Geometry check sheet. Reference: the model listing, model coordinates, mm. Face numbers are marked on the shaded views. A direction names the side the tool comes from. Coordinates: 2 decimals unless noted, no trailing zeros. Loops run counter-clockwise (first coordinate to the right, second up) from the corner with the lowest first, then second, coordinate; pieces in that order, holes last.
from build123d import *

# Parameters (mm, degrees)
MAIN_BODY_DEPTH          = 6.35
BATTERY_SPACING_DEPTH    = 2.54
SKETCH8_R                = 4.064
LIGHT_SOCKETS_DEPTH      = 12.7
LIGHT_LEADS_POCKET_DEPTH = 6.35
WIRE_TRAIL_DEPTH         = 2.54
LEAD_ROOM_DEPTH          = 7.62
FILLET1_R                = 7.62
TAB_SLOTS_DEPTH          = 1.778
SKETCH14_W               = 10.16
SKETCH14_H               = 6.35
SCREW_MOUNT_DEPTH        = 10.16


# Sheet-metal steps are written as plain solids
with BuildPart() as part:
    # Sketch1 → Main Body (new body)
    with BuildSketch(Plane.XY):
        Polygon((-53.975, 0), (53.975, 0), (57.15, 82.161327118), (101.6, 101.6), (101.6, 146.05), (-101.6, 146.05), (-101.6, 101.6), (-57.15, 82.161327118), align=None)
    extrude(amount=-MAIN_BODY_DEPTH)

    # Sketch7 → Battery Spacing (cut)
    with BuildSketch(Plane.XY):
        Polygon((-50.564894027, 76.2), (-47.86564661, 6.35), (47.86564661, 6.35), (50.564894027, 76.2), align=None)
    extrude(amount=-BATTERY_SPACING_DEPTH, mode=Mode.SUBTRACT)

    # Sketch8 → Light Sockets (cut)
    with BuildSketch(Plane.XY):
        with Locations((85.852, 123.825)):
            Circle(SKETCH8_R)
        with Locations((-85.852, 123.825)):
            Circle(SKETCH8_R)
        with BuildLine():
            Line((-5.969, 131.318), (5.969, 131.318))
            ThreePointArc((5.969, 131.318), (13.462, 123.825), (5.969, 116.332))
            Line((5.969, 116.332), (-5.969, 116.332))
            ThreePointArc((-5.969, 116.332), (-13.462, 123.825), (-5.969, 131.318))
        make_face()
    extrude(amount=-LIGHT_SOCKETS_DEPTH, mode=Mode.SUBTRACT)

    # Sketch9 → Light Leads Pocket (add)
    with BuildSketch(Plane(origin=(0, 0, -6.35), x_dir=(-1, 0, 0), z_dir=(0, 0, -1))):
        with BuildLine():
            Line((-9.525, 111.765348554), (-9.525, 99.065348554))
            Line((-9.525, 99.065348554), (9.525, 99.065348554))
            Line((9.525, 99.065348554), (9.525, 111.765348554))
            ThreePointArc((9.525, 111.765348554), (18.413001098, 125.621431375), (5.969, 136.398))
            Line((5.969, 136.398), (-5.969, 136.398))
            ThreePointArc((-5.969, 136.398), (-18.413001098, 125.621431375), (-9.525, 111.765348554))
        make_face()
    extrude(amount=LIGHT_LEADS_POCKET_DEPTH)

    # Sketch10 → Wire Trail (cut)
    with BuildSketch(Plane.XY):
        Polygon((-3.175, 116.332), (3.175, 116.332), (3.175, 76.2), (3.175, 6.35), (3.175, 0), (-3.175, 0), align=None)
    extrude(amount=-WIRE_TRAIL_DEPTH, mode=Mode.SUBTRACT)

    # Sketch12 → Lead Room (cut)
    with BuildSketch(Plane.XY.offset(-2.54)):
        with BuildLine():
            Line((-3.175, 116.332), (-5.960094489, 116.332))
            ThreePointArc((-5.960094489, 116.332), (-13.36178344, 123.73368895), (-5.960094489, 131.135377901))
            Line((-5.960094489, 131.135377901), (6.000168296, 131.135377901))
            ThreePointArc((6.000168296, 131.135377901), (13.401857247, 123.73368895), (6.000168296, 116.332))
            Line((6.000168296, 116.332), (3.175, 116.332))
            Line((3.175, 116.332), (3.175, 103.730451358))
            Line((3.175, 103.730451358), (-3.175, 103.730451358))
            Line((-3.175, 103.730451358), (-3.175, 116.332))
        make_face()
    extrude(amount=-LEAD_ROOM_DEPTH, mode=Mode.SUBTRACT)

    # Fillet1
    fillet1_edges = [part.edges().sort_by_distance(p)[0] for p in [
        (0, 103.730451358, -2.54),
    ]]
    fillet(fillet1_edges, radius=FILLET1_R - 0.0001)  # a hair under: the kernel refuses the full size

    # Sketch13 → Tab Slots (cut)
    with BuildSketch(Plane.XY):
        with BuildLine():
            Line((72.263, 146.05), (72.263, 123.825))
            ThreePointArc((72.263, 123.825), (85.852, 110.236), (99.441, 123.825))
            Line((99.441, 123.825), (99.441, 146.05))
            Line((99.441, 146.05), (72.263, 146.05))
        make_face()
    tab_slots = extrude(amount=-TAB_SLOTS_DEPTH, mode=Mode.SUBTRACT)

    # Mirror1: Tab Slots across plane
    add(tab_slots.mirror(Plane(origin=(0, 0, 0), x_dir=(0, 0, 1), z_dir=(1, 0, 0))), mode=Mode.SUBTRACT)

    # Sketch14 → Screw Mount (add)
    with BuildSketch(Plane.XZ):
        with Locations((48.895, -3.175)):
            Rectangle(SKETCH14_W, SKETCH14_H)
    screw_mount = extrude(amount=SCREW_MOUNT_DEPTH)

    # Mirror2: Screw Mount across plane
    add(screw_mount.mirror(Plane(origin=(0, 0, 0), x_dir=(0, 0, 1), z_dir=(1, 0, 0))))


solid = part.part
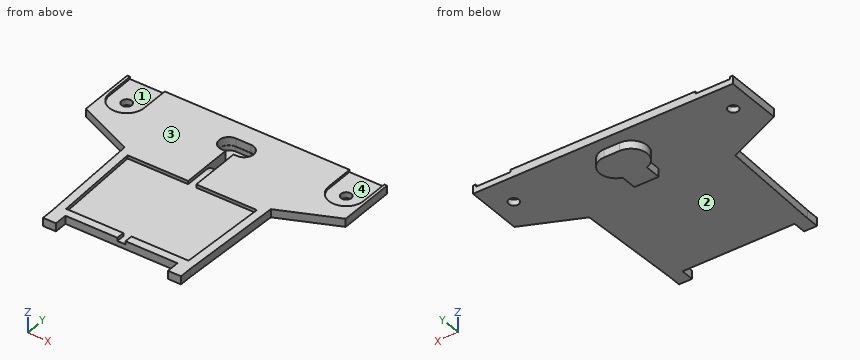
(1) Sectioned sample at C-C on x = -87. Record the cut outline in (y, z), and give its area (3 significant figures).
Findings:
outline: (95.22, -6.35) - (119.93, -6.35) - (119.93, -1.78) - (110.28, -1.78) - (110.28, 0) - (95.22, 0) - close; (127.72, -6.35) - (146.05, -6.35) - (146.05, -1.78) - (127.72, -1.78) - close
area: 224 mm2
(2) Sectioned sample at D-D on x = -24. Record the cut outline in (y, z).
Findings:
outline: (0, -6.35) - (146.05, -6.35) - (146.05, 0) - (76.2, 0) - (76.2, -2.54) - (6.35, -2.54) - (6.35, 0) - (0, 0) - close
(3) Draft check along X on the marked faces 1 and 2. Enter one of: +X half, -X half, draft (parallel to the pull), parting line (faces both ways), or undercut.
Findings:
face 1: undercut
face 2: draft
(4) Scan lines: L1, parallel to X at y = 127, z = -3; L2, parallel to Z at x = 7, y = 125; L3, parallel to X at y = 116, z = -9.25 (3 decimals). Record each from-to range of solid material in increasing order.
Findings:
L1: x = -101.6 to -88.39, -83.32 to -12.76, 12.76 to 83.32, 88.39 to 101.6
L2: z = -12.7 to -10.16
L3: x = -15.81 to -3.175, 3.175 to 15.81
(5) Sectioned sample at B-B on y = 34. Record the cut outline in (x, z).
Findings:
outline: (-55.29, -6.35) - (55.29, -6.35) - (55.29, 0) - (48.93, 0) - (48.93, -2.54) - (-48.93, -2.54) - (-48.93, 0) - (-55.29, 0) - close
(6) Gauge pin test, flat ends, axial feed: pin 1 Ø4 at (y, z) = (6.5, -2.5) entering from +X; pin 2 Ø2 at (x, y) = (-6.5, 21.5) entering from +Z; pin 3 Ø7 at (y, z) = (-4, -2) entering from +X (3 decimals). Record the tip position at first contact, or that the pin passes through.
Findings:
pin 1: stops at x = 54.3
pin 2: stops at z = -2.54
pin 3: stops at x = 53.975
(7) Access from +Z, -Z, +X, -X, +Y, -Y to the whole of each face (thin tool, end or side, straight path). Record for the marked faces 3 and 4.
Findings:
face 3: +Z, +X, -X, +Y, -Y
face 4: +Z, +Y
